from build123d import *

# Parameters (mm, degrees)
SKETCH1_W           = 34
SKETCH1_H           = 28
SKETCH1_W_2         = 28
SKETCH1_H_2         = 22
BOSS_EXTRUDE1_DEPTH = 35
SKETCH2_W           = 8
SKETCH2_H           = 8
CUT_EXTRUDE1_DEPTH  = 35
SKETCH3_W           = 34
SKETCH3_H           = 4
BOSS_EXTRUDE2_DEPTH = 12
SKETCH4_W           = 34
SKETCH4_H           = 4
BOSS_EXTRUDE3_DEPTH = 12
CHAMFER1_SIZE       = 4
SKETCH5_R           = 2
CUT_EXTRUDE2_DEPTH  = 4


with BuildPart() as part:
    # Sketch1 → Boss-Extrude1 (new body)
    with BuildSketch(Plane(origin=(0, 0, 0), x_dir=(1, 0, 0), z_dir=(0, 1, 0))):
        Rectangle(SKETCH1_W, SKETCH1_H)
        Rectangle(SKETCH1_W_2, SKETCH1_H_2, mode=Mode.SUBTRACT)
    extrude(amount=BOSS_EXTRUDE1_DEPTH)

    # Sketch2 → Cut-Extrude1 (cut)
    with BuildSketch(Plane.ZY.offset(17)):
        with Locations((3, 4)):
            Rectangle(SKETCH2_W, SKETCH2_H)
    extrude(amount=-CUT_EXTRUDE1_DEPTH, mode=Mode.SUBTRACT)

    # Sketch3 → Boss-Extrude2 (add)
    with BuildSketch(Plane.XY.offset(14)):
        with Locations((0, 2)):
            Rectangle(SKETCH3_W, SKETCH3_H)
    extrude(amount=BOSS_EXTRUDE2_DEPTH)

    # Sketch4 → Boss-Extrude3 (add)
    with BuildSketch(Plane(origin=(0, 0, -14), x_dir=(-1, 0, 0), z_dir=(0, 0, -1))):
        with Locations((0, 2)):
            Rectangle(SKETCH4_W, SKETCH4_H)
    extrude(amount=BOSS_EXTRUDE3_DEPTH)

    # Chamfer1
    chamfer1_edges = [part.edges().sort_by_distance(p)[0] for p in [
        (-17, 2, 26),
        (17, 2, 26),
        (17, 2, -26),
        (-17, 2, -26),
    ]]
    chamfer(chamfer1_edges, length=CHAMFER1_SIZE)

    # Sketch5 → Cut-Extrude2 (cut)
    with BuildSketch(Plane(origin=(0, 4, 0), x_dir=(1, 0, 0), z_dir=(0, 1, 0))):
        with Locations((-11, -20)):
            Circle(SKETCH5_R)
        with Locations((11, -20)):
            Circle(SKETCH5_R)
        with Locations((-11, 20)):
            Circle(SKETCH5_R)
        with Locations((11, 20)):
            Circle(SKETCH5_R)
    extrude(amount=-CUT_EXTRUDE2_DEPTH, mode=Mode.SUBTRACT)


solid = part.part
The listing builds one solid part. Answer for the finished solid, in the listing's coordinates (mm). A direction names the side the tool comes from. Coordinates: 2 decimals unless noted, no trailing zeros. Write each loop counter-clockwise with the first axis right and the second up, starting at its lowest first coordinate (ties: lowest second). Pieces come first, ordered by that corner, then holes. Notation, with made-up numbers: (34, 9.25) - (81, 9.25) arc R16 cw to (81, 26.25) - close; hole circle Ø9 at (-16.5, 4.5). An arc over 180 degrees is marked (long way). Put each result on its own line as item: value.
1. The part is cut by section A-A on x = -11. Give the vertices of the cut face in (y, z), plus the area to 3 significant figures.
Answer sheet:
outline: (0, -26) - (4, -26) - (4, -22) - (0, -22) - close; (0, -18) - (4, -18) - (4, -14) - (35, -14) - (35, -11) - (0, -11) - close; (0, 11) - (35, 11) - (35, 14) - (4, 14) - (4, 18) - (0, 18) - close; (0, 22) - (4, 22) - (4, 26) - (0, 26) - close
area: 274 mm^2
2. Flat-ended cylindrical pins translate along their axes: pin 1 Ø10 at (x, y) = (3.5, 18) entering from +Z; pin 2 Ø12 at (y, z) = (6.5, -15) entering from -X; pin 3 Ø3.5 at (x, y) = (15.5, 4.5) entering from -Z; pin 4 Ø8 at (x, y) = (12, 19) entering from -Z. Find the tip coordinate at first contact, or state that the pin passes through.
Answer sheet:
pin 1: stops at z = 14
pin 2: stops at x = -17
pin 3: stops at z = -25.18
pin 4: stops at z = -14
3. Find the intervals of material crossed by line 1 along Z through (x, y) = (11, 1.85); line 2 along X through (y, z) = (2.45, -20); line 3 along Z through (x, y) = (-10, 33.5), in increasing order. Write a range as from..to.
Answer sheet:
line 1: z = -26..-22, -18..-11, 11..18, 22..26
line 2: x = -17..-13, -9..9, 13..17
line 3: z = -14..-11, 11..14
4. The part is cut by section B-B on y = 5. Give the vertices of the cut face in (x, z), plus the area to 3 significant figures.
Answer sheet:
outline: (-17, -14) - (17, -14) - (17, -1) - (14, -1) - (14, -11) - (-14, -11) - (-14, -1) - (-17, -1) - close; (-17, 7) - (-14, 7) - (-14, 11) - (14, 11) - (14, 7) - (17, 7) - (17, 14) - (-17, 14) - close
area: 288 mm^2
5. The part is cut by section C-C on x = -1. Give the vertices of the cut face in (y, z).
Answer sheet:
outline: (0, -26) - (4, -26) - (4, -14) - (35, -14) - (35, -11) - (0, -11) - close; (0, 11) - (35, 11) - (35, 14) - (4, 14) - (4, 26) - (0, 26) - close
6. The part is cut by section D-D on z = 20. Give the vertices of the cut face in (x, y).
Answer sheet:
outline: (-17, 0) - (-13, 0) - (-13, 4) - (-17, 4) - close; (-9, 0) - (9, 0) - (9, 4) - (-9, 4) - close; (13, 0) - (17, 0) - (17, 4) - (13, 4) - close
7. Determine the mould class of faces 1 (the face through (15, 2, 24)), 2 (the face through (0, 35, 12)), 3 (the face through (0, 17, -11)), 4 (the face through (-17, 17, 0)) for opening direction X: pulls with the +X half, pulls with the -X half, needs draft (parallel to the pull), parting line crosses it, or undercut.
Answer sheet:
face 1: pulls with the +X half
face 2: needs draft
face 3: undercut
face 4: pulls with the -X half
8. A tool of negligible diameter and unlimited length cuts with its end or side. For faces 5 (the face through (0, 19, -14)), 6 (the face through (0, 0, -16)), 7 (the face through (0, 19, 14)), 8 (the face through (14, 17, 0)), 9 (the face through (15, 8, 3)), from which of +Z, -Z, +X, -X, +Y, -Y can it reach the whole face along a straight path? Write none if from no direction.
Answer sheet:
face 5: -Z, +X, -X, +Y
face 6: +Z, -Z, +X, -X, -Y
face 7: +Z, +X, -X, +Y
face 8: +Y, -Y
face 9: +X, -X, -Y
